Drawing for the job (mm, zero at the part's lowest x, y, z). A direction names the side the tool comes from. Round coordinates to 2 decimals unless told otherwise and drop trailing zeros. Write each loop counter-clockwise with the first axis right and the second up, starting at its lowest first coordinate (ties: lowest second). Pieces come first, ordered by that corner, then holes. Notation, with made-up numbers: M -2.75,-8.75 L 19.25,-8.75 A17 ccw 19.25,5.25 Z; hole C -14,-31 d6. An arc over 180 degrees is marked long. Use a Markdown table: item, result. Add a question column.
1) Wall check: probe 1 along Z at (x, y) = (4.5, 1.85); probe 2 along Z at (x, y) = (3.75, 1.2); probe 3 along Y at (x, z) = (5, 2.75). Give the ranges that are in metal, low to high.
2) Which spindle directions (+Z, -Z, +X, -X, +Y, -Y) get a long thin tool onto all of the face, cutting with end or side? Do the marked faces 1 and 2. Say none if no direction does.
3) Slice it at B-B on x = 4.5. Write the cut outline in (y, z).
4) Slice it at C-C on y = 1.15. Write the cut outline in (x, z), plus the area to 3 significant figures.
5) Slice it at A-A on z = 4.5. Write the cut outline in (x, y).
6) Two-plate mould, pull along Z, no slides. Class the marked faces 3, 4 and 5: released by +Z, released by -Z, zero draft, split by the parting line, or undercut.
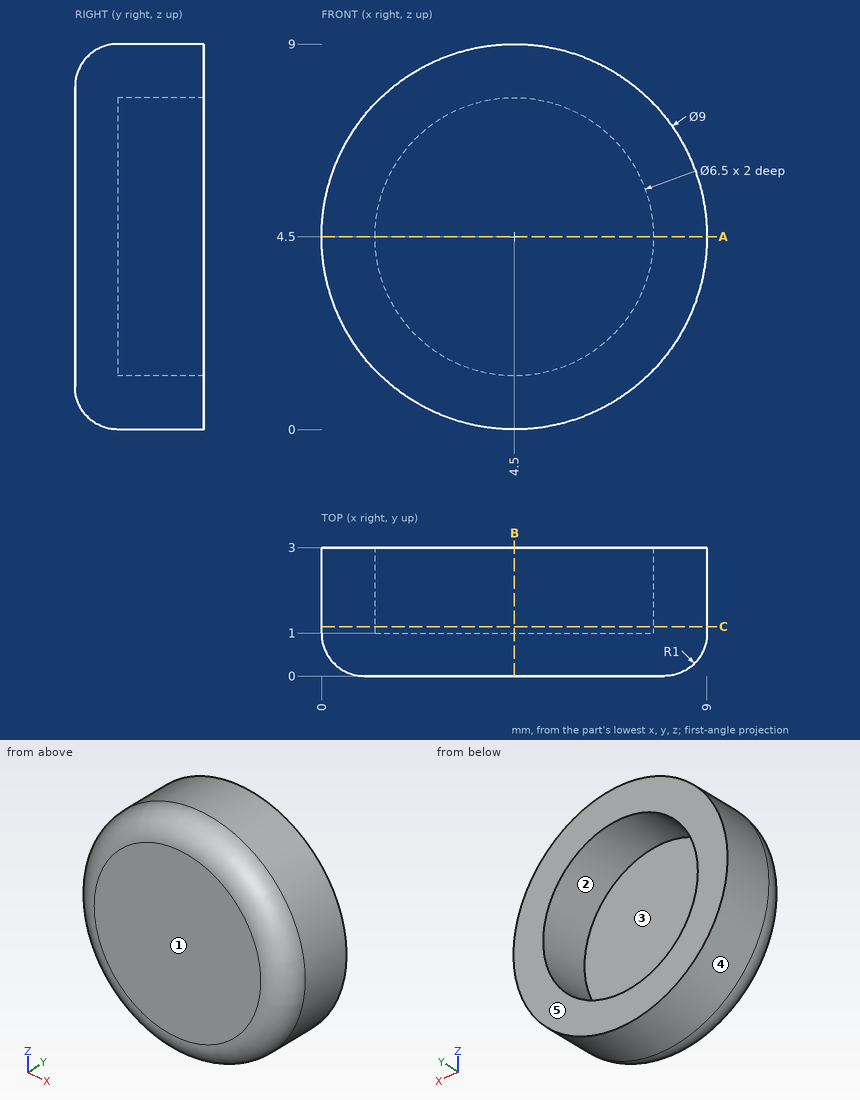
Entries:
| question | item | result |
|---|---|---|
| 1 | probe 1 | z = 0 to 1.25, 7.75 to 9 |
| 1 | probe 2 | z = 0.06 to 1.34, 7.66 to 8.94 |
| 1 | probe 3 | y = 0 to 1 |
| 2 | face 1 | +Z, -Z, +X, -X, -Y |
| 2 | face 2 | +Y |
| 3 | outline | M 0,1 A1 ccw 1,0 L 3,0 L 3,1.25 L 1,1.25 L 1,7.75 L 3,7.75 L 3,9 L 1,9 A1 ccw 0,8 Z |
| 4 | outline | C 4.5,4.5 d9; hole C 4.5,4.5 d6.5 |
| 4 | area | 30.4 mm^2 |
| 5 | outline | M 0,1 A1 ccw 1,0 L 8,0 A1 ccw 9,1 L 9,3 L 7.75,3 L 7.75,1 L 1.25,1 L 1.25,3 L 0,3 Z |
| 6 | face 3 | undercut |
| 6 | face 4 | split by the parting line |
| 6 | face 5 | zero draft |
